For this review, take the finished solid that the model builds, in its own axes (mm). Give positions to 0.01 mm unless a question says otherwise; leave off trailing zeros. Order: outer loops, then holes, each group sorted by start corner. A loop starts at its lowest first (then second) coordinate and runs counter-clockwise, first axis right, second up. Notation, with made-up numbers: (51.25, 42.25) - (88.25, 42.25) arc R13 cw to (88.25, 51.25) - close; hole circle Ø2 at (84.25, -23.75). An arc over 180 degrees is marked (long way). Put each result on its own line as item: value. Start each with the question number.
```python
from build123d import *

# Parameters (mm, degrees)
BOSS_EXTRUDE1_DEPTH = 5.08
SKETCH2_R           = 1.7272
CUT_EXTRUDE1_DEPTH  = 5.08


with BuildPart() as part:
    # Sketch1 → Boss-Extrude1 (new body)
    with BuildSketch(Plane.XY):
        with BuildLine():
            Line((-15.343524861, 23.838622958), (0, 0))
            Line((0, 0), (56.065565283, 36.086119416))
            Line((56.065565283, 36.086119416), (64.573765087, 69.628973221))
            ThreePointArc((64.573765087, 69.628973221), (19.853616616, 55.043986881), (-15.343524861, 23.838622958))
        make_face()
    extrude(amount=BOSS_EXTRUDE1_DEPTH)

    # Sketch2 → Cut-Extrude1 (cut)
    with BuildSketch(Plane.XY.offset(5.08)):
        with Locations((46.012387455, 35.57370741)):
            Circle(SKETCH2_R)
        with Locations((-1.023333215, 17.191896262)):
            Circle(SKETCH2_R)
        with Locations((4.388908167, 8.783112568)):
            Circle(SKETCH2_R)
        with Locations((40.600146073, 43.982491105)):
            Circle(SKETCH2_R)
        Polygon((10.799924344, 6.773067648), (45.186804384, 28.905887557), (34.189129896, 45.992536024), (-0.197750144, 23.859716115), align=None)
    extrude(amount=-CUT_EXTRUDE1_DEPTH, mode=Mode.SUBTRACT)


solid = part.part
```
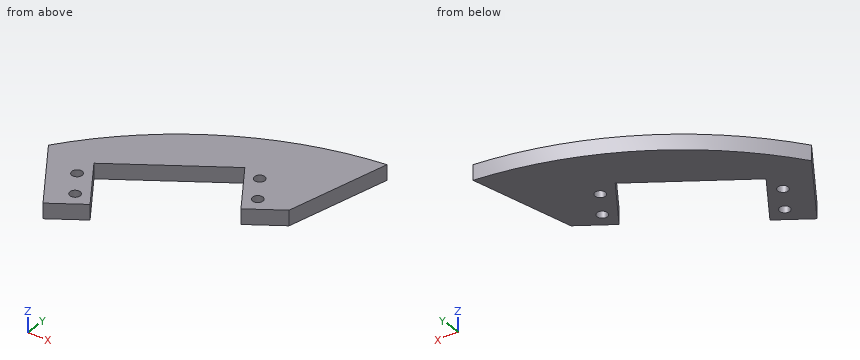
1. Wall thickness on line 1 (X direction, y = 43.5, z = 3.9); line 2 (X direction, y = 30, z = 4.25); line 3 (Y direction, x = 45.5, z = 0.45): over which ranges is each line inside the solid? List them lowest first. Write a range as from..to.
2. Add section D-D, the plane y = 62.5. Give the boundary of the cut face in (x, z).
3. Add section A-A, the plane z = 4.15. Give the boundary of the cut face in (x, y).
4. Clearance check with flat-ended pins moving along their axes: pin 1 (3 mm diameter, centred on x = 46.01, y = 35.57, fed in from +Z); pin 2 (2 mm diameter, centred on x = 15, y = 50.5, fed in from -Z); pin 3 (1.5 mm diameter, centred on x = 54.5, z = 1.5, fed in from -Y); pin 4 (3 mm diameter, centred on x = -2, z = 0.5, fed in from +Y). State where each tip first meets the part, or that it passes through.
5. Add section B-B, the plane y = 39.5. Give the boundary of the cut face in (x, z), then the cut area to 3 significant figures.
6. Add section C-C, the plane x = 31.5. Give the boundary of the cut face in (y, z).
Found:
1. line 1: x = 3.26..30.32, 35.79..38.94, 42.26..57.95
1. line 2: x = -10.42..9.34, 44.48..46.61
1. line 3: y = 29.29..33.92, 37.22..65.87
2. outline: (35.48, 0) - (62.77, 0) - (62.77, 5.08) - (35.48, 5.08) - close
3. outline: (-15.34, 23.84) - (0, 0) - (10.72, 6.9) - (-0.2, 23.86) - (34.19, 45.99) - (45.11, 29.03) - (56.07, 36.09) - (64.57, 69.63) arc R115.51 ccw to start; hole circle Ø3.45 at (-1.02, 17.19); hole circle Ø3.45 at (4.39, 8.78); hole circle Ø3.45 at (40.6, 43.98); hole circle Ø3.45 at (46.01, 35.57)
4. pin 1: passes through
4. pin 2: stops at z = 0
4. pin 3: stops at y = 34.6
4. pin 4: stops at y = 40.22
5. outline: (-1.28, 0) - (24.1, 0) - (24.1, 5.08) - (-1.28, 5.08) - close; (38.37, 0) - (56.93, 0) - (56.93, 5.08) - (38.37, 5.08) - close
5. area: 223 mm^2
6. outline: (44.26, 0) - (60.87, 0) - (60.87, 5.08) - (44.26, 5.08) - close
